Could you check a few things on this model? Use its own coordinates, in mm. Round coordinates to 2 decimals unless told otherwise and drop trailing zeros. Loops run counter-clockwise (first coordinate to the right, second up) from the corner with the lowest first, then second, coordinate; pieces in that order, holes last.
Autodesk Inventor part; units mm, degrees
ref_plane "YZ Plane" through (0, 0, 0) normal (1, 0, 0) x (0, 1, 0)
ref_plane "XZ Plane" through (0, 0, 0) normal (0, 1, 0) x (-1, 0, 0)
ref_plane "XY Plane" through (0, 0, 0) normal (0, 0, 1) x (1, 0, 0)
sketch "Sketch1" plane through (0, 0, 0) normal (0, 0, 1) x (1, 0, 0)
  line L0 (-82.5, 3) -> (-82.5, 18) construction
  line L1 (82.5, 3) -> (-82.5, 3) construction
  line L2 (-51, 0) -> (-51, 3) construction
  line L3 (-82.5, 0) -> (-82.5, -10)
  line L4 (-82.5, -10) -> (0, -10)
  line L5 (0, -10) -> (0, 0)
  line L6 (0, 0) -> (-82.5, 0)
  dimension "d0" = 10
revolve "Revolution1" add sketch "Sketch1" angle 360 about axis through (0, -10, 0) along (0, 1, 0)
sketch "Sketch2" plane through (0, -10, 0) normal (0, -1, 0) x (1, 0, 0)
  circle A0 centre (0, 0) radius 49.3853 construction
  circle A1 centre (-62.5, 0) radius 9.2
  circle A2 centre (0, 62.5) radius 9.2
  circle A3 centre (0, 0) radius 82.3
  circle A4 centre (62.5, 0) radius 9.2
  circle A5 centre (0, -62.5) radius 9.2
  point P0 (0, 0)
  point P1 (62.5, 0)
hole "Hole1" at (62.5, -10, 0) direction (0, 1, 0) diameter 18 end through all
pattern_circular "Circular Pattern1" count 4 over 360 about axis through (0, -10, 0) along (0, 1, 0) of "Hole1"
properties part number "vakkarima2" material "Steel, Alloy"
Item 1: If we section it at D-D, the plane y = -2: Please give me the cut outline in (x, z).
Results list:
outline: circle Ø165 at (0, 0); hole circle Ø18 at (-62.5, 0); hole circle Ø18 at (0, -62.5); hole circle Ø18 at (0, 62.5); hole circle Ø18 at (62.5, 0)
Item 2: If we section it at C-C, the plane x = 62.5: Please give me the cut outline in (y, z).
Results list:
outline: (-10, -53.85) - (0, -53.85) - (0, -9) - (-10, -9) - close; (-10, 9) - (0, 9) - (0, 53.85) - (-10, 53.85) - close
Item 3: If we section it at A-A, the plane x = 0: Please give me the cut outline in (y, z).
Results list:
outline: (-10, -82.5) - (0, -82.5) - (0, -71.5) - (-10, -71.5) - close; (-10, -53.5) - (0, -53.5) - (0, 53.5) - (-10, 53.5) - close; (-10, 71.5) - (0, 71.5) - (0, 82.5) - (-10, 82.5) - close
Item 4: If we section it at B-B, the plane z = -7: Please give me the cut outline in (x, y).
Results list:
outline: (-82.2, -10) - (-68.16, -10) - (-68.16, 0) - (-82.2, 0) - close; (-56.84, -10) - (56.84, -10) - (56.84, 0) - (-56.84, 0) - close; (68.16, -10) - (82.2, -10) - (82.2, 0) - (68.16, 0) - close
Item 5: If I drill on line 1 along X through (y, z) = (-0.5, -0.5); line 2 along X through (y, z) = (-3.75, -8); line 3 along X through (y, z) = (-6, 69), over which ranges is the centre line in solid material (lowest first)?
Results list:
line 1: x = -82.5 to -71.49, -53.51 to 53.51, 71.49 to 82.5
line 2: x = -82.11 to -66.62, -58.38 to 58.38, 66.62 to 82.11
line 3: x = -45.22 to -6.22, 6.22 to 45.22
Item 6: We'd pull the mould along Z, two halves only. Please class faces 1 (the cylindrical face through (-1.951, -4.93, 71.286)), 2 (the cylindrical face through (17.88, -5.07, 80.54)), 3 (the flat face through (1, -10, 1)): released by +Z, released by -Z, zero draft, split by the parting line, or undercut.
Results list:
face 1: undercut
face 2: split by the parting line
face 3: zero draft
Item 7: Will these pins go through, and if not, where does the flat tip stop? pin 1 (16 mm diameter, centred on x = 62.5, z = 0, fed in from +Y); pin 2 (1.5 mm diameter, centred on y = -4, z = 4.5, fed in from -X); pin 3 (4 mm diameter, centred on x = 32.5, y = -6, fed in from -Z); pin 4 (2 mm diameter, centred on x = -16, y = -2, fed in from +Z).
Results list:
pin 1: passes through
pin 2: stops at x = -82.41
pin 3: stops at z = -76.66
pin 4: stops at z = 81.12
